Part model, mm, in its own coordinate system. Give positions to 0.01 mm unless a question says otherwise; leave off trailing zeros. Order: outer loops, then holes, each group sorted by start corner. A loop starts at its lowest first (then second) coordinate and runs counter-clockwise, first axis right, second up. Notation, with made-up numbers: (71, -28.5) - (116, -28.5) arc R28 ccw to (116, 5.5) - close; hole circle Ø1 at (69, 76). An arc over 180 degrees is marked (long way). One line per item, written item: value.
```python
from build123d import *

# Parameters (mm, degrees)
SALIENTE_EXTRUIR1_DEPTH = 36
REDONDEO2_R             = 0.4


with BuildPart() as part:
    # Croquis1 → Saliente-Extruir1 (new body)
    with BuildSketch(Plane.XY):
        with BuildLine():
            Line((0.8, 2.209637979), (0.8, 0.8))
            Line((0.8, 0.8), (2.209637979, 0.8))
            ThreePointArc((2.209637979, 0.8), (2.35, 0), (2.209637979, -0.8))
            Line((2.209637979, -0.8), (0.8, -0.8))
            Line((0.8, -0.8), (0.8, -2.209637979))
            ThreePointArc((0.8, -2.209637979), (0, -2.35), (-0.8, -2.209637979))
            Line((-0.8, -2.209637979), (-0.8, -0.8))
            Line((-0.8, -0.8), (-2.209637979, -0.8))
            ThreePointArc((-2.209637979, -0.8), (-2.35, 0), (-2.209637979, 0.8))
            Line((-2.209637979, 0.8), (-0.8, 0.8))
            Line((-0.8, 0.8), (-0.8, 2.209637979))
            ThreePointArc((-0.8, 2.209637979), (0, 2.35), (0.8, 2.209637979))
        make_face()
    extrude(amount=SALIENTE_EXTRUIR1_DEPTH)

    # Redondeo2
    redondeo2_edges = [part.edges().sort_by_distance(p)[0] for p in [
        (2.35, 0, 0),
        (0, -2.35, 0),
        (-2.35, 0, 0),
        (0, 2.35, 0),
        (-2.35, 0, 36),
        (0, -2.35, 36),
        (2.35, 0, 36),
        (0, 2.35, 36),
    ]]
    fillet(redondeo2_edges, radius=REDONDEO2_R)


solid = part.part
```
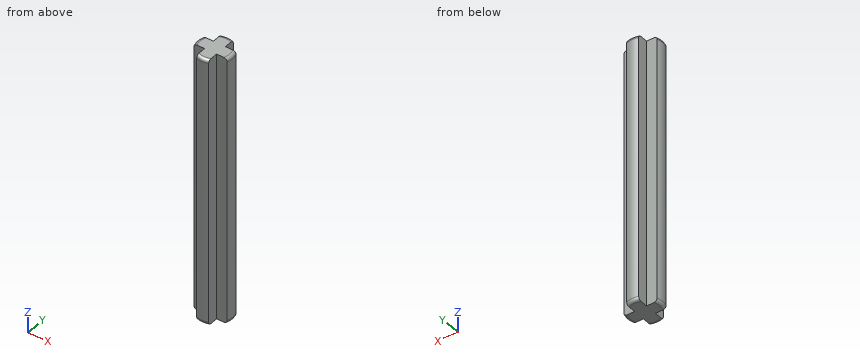
1) Slice it at B-B on x = 1.25. Write the cut outline in (y, z).
Answer:
outline: (-0.8, 0) - (0.8, 0) - (0.8, 36) - (-0.8, 36) - close
2) Wall check: line 1 along X through (y, z) = (1.2, 15); line 2 along Y through (x, z) = (0.15, 7). Give the ranges that are in metal, low to high. Write a range as [from, to].
Answer:
line 1: x = [-0.8, 0.8]
line 2: y = [-2.35, 2.35]
3) Drop flat-ended pins along their axis: P1, Ø0.7, axis at x = 1.5, z = 21, coming from the +Y side; P2, Ø1.6, axis at x = 2, z = 16.5, coming from the -Y side; P3, Ø1.6, axis at y = -1.5, z = 14, coming from the -X side. Give the stop position or say it passes through.
Answer:
P1: stops at y = 0.8
P2: stops at y = -0.8
P3: stops at x = -2.24
4) Slice it at A-A on z = 20.5. Write the cut outline in (x, y), then the cut area to 3 significant figures.
Answer:
outline: (-2.21, -0.8) - (-0.8, -0.8) - (-0.8, -2.21) arc R2.35 ccw to (0.8, -2.21) - (0.8, -0.8) - (2.21, -0.8) arc R2.35 ccw to (2.21, 0.8) - (0.8, 0.8) - (0.8, 2.21) arc R2.35 ccw to (-0.8, 2.21) - (-0.8, 0.8) - (-2.21, 0.8) arc R2.35 ccw to start
area: 12.2 mm2
